from build123d import *

# Parameters (mm, degrees)
BOSS_EXTRUDE4_DEPTH = 2
BOSS_EXTRUDE7_DEPTH = 25
BOSS_EXTRUDE8_DEPTH = 11.5
CUT_EXTRUDE4_DEPTH  = 2
CUT_EXTRUDE5_DEPTH  = 2
CUT_EXTRUDE6_DEPTH  = 2
CHAMFER2_SIZE       = 1
CUT_EXTRUDE8_REACH  = 74.555


with BuildPart() as part:
    # Sketch8 → Boss-Extrude4 (new body)
    with BuildSketch(Plane(origin=(0, 0, 0), x_dir=(1, 0, 0), z_dir=(0, 1, 0))):
        Polygon((19.761418396, 5.799677564), (27.278959362, 8.535838711), (29.331080222, 2.897682986), (15.874806811, -2), (-15.874806811, -2), (-39.501605359, 6.599451403), (-36.081403926, 15.996377611), (-30.443248201, 13.944256751), (-33.179409348, 6.426715784), (-15.522152849, 0), (15.522152849, 0), (17.975516043, 0.892951176), align=None)
    extrude(amount=BOSS_EXTRUDE4_DEPTH)

    # Sketch12 → Boss-Extrude7 (add)
    with BuildSketch(Plane.XZ):
        Polygon((-39.501605359, -6.599451403), (-15.874806811, 2), (15.874806811, 2), (29.331080222, -2.897682986), (28.647039935, -4.777068227), (17.975516043, -0.892951176), (15.522152849, 0), (-15.522152849, 0), (-33.179409348, -6.426715784), (-38.817565073, -8.478836644), align=None)
    extrude(amount=BOSS_EXTRUDE7_DEPTH)

    # Sketch13 → Boss-Extrude8 (add)
    with BuildSketch(Plane.XZ):
        Polygon((-34.202018685, -15.312337324), (-36.081403926, -15.996377611), (-38.133524786, -10.358221886), (-36.254139544, -9.674181599), align=None)
        Polygon((-32.322633443, -14.628297037), (-30.443248201, -13.944256751), (-33.179409348, -6.426715784), (-35.05879459, -7.110756071), align=None)
        Polygon((19.761418396, -5.799677564), (27.278959362, -8.535838711), (27.962999649, -6.656453469), (18.868467219, -3.34631437), align=None)
    extrude(amount=BOSS_EXTRUDE8_DEPTH)

    # Sketch15 → Cut-Extrude4 (cut)
    with BuildSketch(Plane(origin=(0.447666384, 0, 1.22995328), x_dir=(-0.9396926207859031, 0, 0.34202014332568326), z_dir=(-0.34202014332568326, 0, -0.9396926207859031))):
        Polygon((-24.553265595, -11.5), (-28.553265595, -4.75), (-28.553265595, -11.5), align=None)
    extrude(amount=-CUT_EXTRUDE4_DEPTH, mode=Mode.SUBTRACT)

    # Sketch16 → Cut-Extrude5 (cut)
    with BuildSketch(Plane(origin=(2.499787244, 0, 6.868109005), x_dir=(0.9396926207859029, 0, -0.3420201433256841), z_dir=(0.34202014332568403, 0, 0.9396926207859028))):
        Polygon((21.393332062, -25), (28.553265595, -11.5), (28.553265595, -25), align=None)
    extrude(amount=-CUT_EXTRUDE5_DEPTH, mode=Mode.SUBTRACT)

    # Sketch17 → Cut-Extrude6 (cut)
    with BuildSketch(Plane(origin=(-2.499787244, 0, 6.868109005), x_dir=(0.9396926207859133, 0, 0.3420201433256553), z_dir=(-0.3420201433256553, 0, 0.9396926207859133))):
        Polygon((-39.37651238, -25), (-39.37651238, -11.5), (-36.37651238, -25), align=None)
    extrude(amount=-CUT_EXTRUDE6_DEPTH, mode=Mode.SUBTRACT)

    # Chamfer2
    chamfer2_edges = [part.edges().sort_by_distance(p)[0] for p in [
        (-37.791504643, 2, -11.297914507),
        (28.305019792, 2, -5.716760848),
    ]]
    chamfer(chamfer2_edges, length=CHAMFER2_SIZE)

    # Cut-Extrude8: up to this face of the body (flat: up to its plane)
    cut_extrude8_end = Plane(part.part.faces().sort_by_distance((-31.811328775, -4.75, -10.185486267))[0])
    # Sketch23 → Cut-Extrude8 (cut, up to the picked face)
    with BuildSketch(Plane(origin=(-37.001818116, 0, -13.467560408), x_dir=(-0.3420201433256551, 0, 0.9396926207859133), z_dir=(-0.9396926207859133, 0, -0.3420201433256551)), mode=Mode.PRIVATE) as cut_extrude8_sk1:
        Polygon((0.308888942, -11.5), (-2.691111058, -5.25), (-2.691111058, -11.5), align=None)
    cut_extrude8_tool1 = split(extrude(cut_extrude8_sk1.sketch, amount=-CUT_EXTRUDE8_REACH, mode=Mode.PRIVATE), bisect_by=cut_extrude8_end, keep=Keep.BOTH, mode=Mode.PRIVATE)
    add(cut_extrude8_tool1.solids().sort_by(Axis((-36.423424, -9.416667, -15.056685), (0.9396926207859133, 0, 0.3420201433256551)))[0], mode=Mode.SUBTRACT)


solid = part.part
Build history of the part. All positions in model axes, mm. A direction names the side the tool comes from. Give positions to 0.01 mm unless a question says otherwise; leave off trailing zeros. Loops run counter-clockwise (first coordinate to the right, second up) from the corner with the lowest first, then second, coordinate; pieces in that order, holes last. Notation, with made-up numbers: (-3.75, -38.75) -> (10.25, -38.75) arc R15 cw to (10.25, -22.75) -> close; hole circle Ø4 at (-39, 11.25). An arc over 180 degrees is marked (long way). Answer in a Markdown table with one row per item.
Item 1: Slice it at A-A on y = -2.5. Write the cut outline in (x, z), plus the area to 3 significant figures.
Findings below:
| item | result |
|---|---|
| outline | (-39.5, -6.6) -> (-38.82, -8.48) -> (-35.06, -7.11) -> (-32.32, -14.63) -> (-30.44, -13.94) -> (-33.18, -6.43) -> (-15.52, 0) -> (15.52, 0) -> (28.65, -4.78) -> (29.33, -2.9) -> (15.87, 2) -> (-15.87, 2) -> close; (-38.13, -10.36) -> (-36.08, -16) -> (-34.2, -15.31) -> (-36.25, -9.67) -> close; (18.87, -3.35) -> (19.76, -5.8) -> (27.28, -8.54) -> (27.96, -6.66) -> close |
| area | 187 mm² |
Item 2: Tool access for faces 1 (the flat face through (-35.5, 0, -11.3)), 2 (the flat face through (0, -11, 0)), 3 (the flat face through (-31.79, -4.84, -10.24)), 4 (the flat face through (-37, -11.5, -11)): list every direction of +Z, -Z, +X, -X, +Y, -Y with a clear straight run to the whole face (end or side of a thin tool).
Findings below:
| item | result |
|---|---|
| face 1 | -Y |
| face 2 | -Z, +Y, -Y |
| face 3 | +Y, -Y |
| face 4 | -Z, +X, -X, -Y |
Item 3: Slice it at C-C on y = -16. Write the cut outline in (x, z), plus the area to 3 significant figures.
Findings below:
| item | result |
|---|---|
| outline | (-38.56, -6.26) -> (-37.88, -8.14) -> (-15.52, 0) -> (15.52, 0) -> (26.4, -3.96) -> (27.09, -2.08) -> (15.87, 2) -> (-15.87, 2) -> close |
| area | 134 mm² |
Item 4: Flat gauge pins, fed straight in: P1, Ø1.1, axis at x = 23, z = -4.5, coming from the -Y side; P2, Ø8, axis at x = 3, y = -8, coming from the -Z side; P3, Ø6, axis at x = -21.5, y = -14, coming from the -Z side. Where does each tip first touch, or does it go through?
Findings below:
| item | result |
|---|---|
| P1 | stops at y = -11.5 |
| P2 | stops at z = 0 |
| P3 | stops at z = -3.27 |
Item 5: Slice it at B-B on x = -12. Write the cut outline in (y, z), plus the area to 3 significant figures.
Findings below:
| item | result |
|---|---|
| outline | (-25, 0) -> (2, 0) -> (2, 2) -> (-25, 2) -> close |
| area | 54.0 mm² |
Item 6: Mould opens along Z. For faces 5 (the flat face through (25.7, -8.2, -6.9)), 6 (the flat face through (-33, -11.5, -9)), 7 (the flat face through (-37.21, -5.67, -10.02)) say: pulls with the +Z half, pulls with the -Z half, needs draft (parallel to the pull), parting line crosses it, or undercut.
Findings below:
| item | result |
|---|---|
| face 5 | pulls with the -Z half |
| face 6 | needs draft |
| face 7 | undercut |
Item 7: Slice it at D-D on y = -6.75. Write the cut outline in (x, z).
Findings below:
| item | result |
|---|---|
| outline | (-39.5, -6.6) -> (-38.82, -8.48) -> (-35.06, -7.11) -> (-32.57, -13.95) -> (-30.69, -13.27) -> (-33.18, -6.43) -> (-15.52, 0) -> (15.52, 0) -> (28.65, -4.78) -> (29.33, -2.9) -> (15.87, 2) -> (-15.87, 2) -> close; (-38.13, -10.36) -> (-36.33, -15.32) -> (-34.45, -14.64) -> (-36.25, -9.67) -> close; (18.87, -3.35) -> (19.76, -5.8) -> (26.17, -8.13) -> (26.85, -6.25) -> close |
Item 8: Probe line 1 along Z through (x, y) = (-1, -19); line 2 along X through (y, z) = (-6.75, -10.5). List the from-to ranges inside material, lowest first. Write a range as [from, to].
Findings below:
| item | result |
|---|---|
| line 1 | z = [0, 2] |
| line 2 | x = [-38.08, -35.95], [-33.83, -31.7] |
